Work out the finished part from the listing and answer in its coordinate system (mm). Round coordinates to 2 decimals unless told otherwise and drop trailing zeros. Order: outer loops, then holes, each group sorted by start corner. A loop starts at its lowest first (then second) coordinate and runs counter-clockwise, first axis right, second up. Notation, with made-up numbers: (68, 59.5) - (78, 59.5) arc R22 cw to (78, 84.5) - close; hole circle Ø5 at (29, -26). An arc over 180 degrees is marked (long way). One line per question, with ' | ' between items. Start each with the question number.
from build123d import *

# Parameters (mm, degrees)
SKETCH1_R                = 26.125
BOSS_EXTRUDE1_DEPTH      = 1
SKETCH2_W                = 0.65
SKETCH2_H                = 3
CUT_EXTRUDE2_DEPTH       = 38.984224
CUT_EXTRUDE2_DEPTH_BACK  = 38.984224
SKETCH3_R                = 23.625
BOSS_EXTRUDE2_DEPTH      = 13
FILLET1_R                = 1
CIRPATTERN1_COUNT        = 6
FILLET1_OF_CIRPATTERN1_R = 1


with BuildPart() as part:
    # Sketch1 → Boss-Extrude1 (new body)
    with BuildSketch(Plane(origin=(0, 0, 0), x_dir=(1, 0, 0), z_dir=(0, 1, 0))):
        with Locations(Location((0, 0, 0), (0, 0, 270))):
            Circle(SKETCH1_R)
    extrude(amount=BOSS_EXTRUDE1_DEPTH)

    # Sketch2 → Revolve1 (revolve)
    with BuildSketch(Plane.XY, mode=Mode.PRIVATE) as revolve1_sk:
        with Locations((26.45, 1.5)):
            Rectangle(SKETCH2_W, SKETCH2_H)
    revolve(revolve1_sk.sketch.rotate(Axis((0, 0, 0), (0, 1, 0)), 90), axis=Axis((0, 0, 0), (0, 1, 0)))

    # Sketch3 → Cut-Extrude2 (cut, two sides: drawn at the far end of the back side and taken through both)
    with BuildSketch(Plane(origin=(0, 0, 0), x_dir=(1, 0, 0), z_dir=(0, 1, 0)).offset(-CUT_EXTRUDE2_DEPTH_BACK)):
        with Locations(Location((0, 0, 0), (0, 0, 270))):
            Circle(SKETCH3_R)
    extrude(amount=CUT_EXTRUDE2_DEPTH + CUT_EXTRUDE2_DEPTH_BACK, mode=Mode.SUBTRACT)

    # Sketch5 → Boss-Extrude2 (add)
    with BuildSketch(Plane(origin=(0, 0, 0), x_dir=(1, 0, 0), z_dir=(0, 1, 0))):
        with BuildLine():
            Line((25.948808, 6.6), (25.318865, 6.439776))
            ThreePointArc((25.318865, 6.439776), (26.125, 0), (25.318865, -6.439776))
            Line((25.318865, -6.439776), (25.948808, -6.6))
            ThreePointArc((25.948808, -6.6), (26.775, 0), (25.948808, 6.6))
        make_face()
    boss_extrude2 = extrude(amount=BOSS_EXTRUDE2_DEPTH)

    # Fillet1
    # the kernel refuses this fillet: 1 mm, written as the material it takes off along each edge
    with BuildSketch(Plane(origin=(0, 13, 0), x_dir=(0.9431839321448116, 0, -0.33227107930701955), z_dir=(-0.33227107930701955, 0, -0.9431839321448116))) as fillet1_piece_1:
        with BuildLine():
            CenterArc((27.125, 0.93675), FILLET1_R, 180, 69.512685)
            Line((26.125, 0.93675), (26.105, 0.93675))
            Line((26.105, 0.93675), (26.105, 0))
            Line((26.105, 0), (26.125, -0.02))
            ThreePointArc((26.125, -0.02), (26.45, -0.02), (26.768, -0.018735))
            Line((26.768, -0.018735), (26.775, 0))
        make_face()
    revolve(axis=Axis((0, 13, 0), (0, -1, 0)), revolution_arc=38.813358, mode=Mode.SUBTRACT)

    # CirPattern1: Boss-Extrude2 ×6 about axis
    cirpattern1_axis = Axis((0, 0, 0), (0, 1, 0))
    for i in range(1, CIRPATTERN1_COUNT):
        add(boss_extrude2.rotate(cirpattern1_axis, i * 360 / CIRPATTERN1_COUNT))

    # Fillet1 of CirPattern1
    # the kernel refuses this fillet: 1 mm, written as the material it takes off along each edge
    with BuildSketch(Plane(origin=(0, 13, 0), x_dir=(0.18383677044965302, 0, -0.9829567853322146), z_dir=(-0.9829567853322146, 0, -0.18383677044965302))) as fillet1_of_cirpattern1_piece_1:
        with BuildLine():
            CenterArc((27.125, 0.93675), FILLET1_OF_CIRPATTERN1_R, 180, 69.512685)
            Line((26.125, 0.93675), (26.105, 0.93675))
            Line((26.105, 0.93675), (26.105, 0))
            Line((26.105, 0), (26.125, -0.02))
            ThreePointArc((26.125, -0.02), (26.45, -0.02), (26.768, -0.018735))
            Line((26.768, -0.018735), (26.775, 0))
        make_face()
    revolve(axis=Axis((0, 13, 0), (0, -1, 0)), revolution_arc=38.813358, mode=Mode.SUBTRACT)
    with BuildSketch(Plane(origin=(0, 13, 0), x_dir=(-0.7593471616951585, 0, -0.6506857060251953), z_dir=(-0.6506857060251953, 0, 0.7593471616951585))) as fillet1_of_cirpattern1_piece_2:
        with BuildLine():
            CenterArc((27.125, 0.93675), FILLET1_OF_CIRPATTERN1_R, 180, 69.512685)
            Line((26.125, 0.93675), (26.105, 0.93675))
            Line((26.105, 0.93675), (26.105, 0))
            Line((26.105, 0), (26.125, -0.02))
            ThreePointArc((26.125, -0.02), (26.45, -0.02), (26.768, -0.018735))
            Line((26.768, -0.018735), (26.775, 0))
        make_face()
    revolve(axis=Axis((0, 13, 0), (0, -1, 0)), revolution_arc=38.813358, mode=Mode.SUBTRACT)
    with BuildSketch(Plane(origin=(0, 13, 0), x_dir=(-0.9431839321448114, 0, 0.3322710793070194), z_dir=(0.3322710793070194, 0, 0.9431839321448114))) as fillet1_of_cirpattern1_piece_3:
        with BuildLine():
            CenterArc((27.125, 0.93675), FILLET1_OF_CIRPATTERN1_R, 180, 69.512685)
            Line((26.125, 0.93675), (26.105, 0.93675))
            Line((26.105, 0.93675), (26.105, 0))
            Line((26.105, 0), (26.125, -0.02))
            ThreePointArc((26.125, -0.02), (26.45, -0.02), (26.768, -0.018735))
            Line((26.768, -0.018735), (26.775, 0))
        make_face()
    revolve(axis=Axis((0, 13, 0), (0, -1, 0)), revolution_arc=38.813358, mode=Mode.SUBTRACT)
    with BuildSketch(Plane(origin=(0, 13, 0), x_dir=(-0.18383677044965369, 0, 0.9829567853322146), z_dir=(0.9829567853322146, 0, 0.18383677044965369))) as fillet1_of_cirpattern1_piece_4:
        with BuildLine():
            CenterArc((27.125, 0.93675), FILLET1_OF_CIRPATTERN1_R, 180, 69.512685)
            Line((26.125, 0.93675), (26.105, 0.93675))
            Line((26.105, 0.93675), (26.105, 0))
            Line((26.105, 0), (26.125, -0.02))
            ThreePointArc((26.125, -0.02), (26.45, -0.02), (26.768, -0.018735))
            Line((26.768, -0.018735), (26.775, 0))
        make_face()
    revolve(axis=Axis((0, 13, 0), (0, -1, 0)), revolution_arc=38.813358, mode=Mode.SUBTRACT)
    with BuildSketch(Plane(origin=(0, 13, 0), x_dir=(0.7593471616951586, 0, 0.6506857060251952), z_dir=(0.6506857060251952, 0, -0.7593471616951586))) as fillet1_of_cirpattern1_piece_5:
        with BuildLine():
            CenterArc((27.125, 0.93675), FILLET1_OF_CIRPATTERN1_R, 180, 69.512685)
            Line((26.125, 0.93675), (26.105, 0.93675))
            Line((26.105, 0.93675), (26.105, 0))
            Line((26.105, 0), (26.125, -0.02))
            ThreePointArc((26.125, -0.02), (26.45, -0.02), (26.768, -0.018735))
            Line((26.768, -0.018735), (26.775, 0))
        make_face()
    revolve(axis=Axis((0, 13, 0), (0, -1, 0)), revolution_arc=38.813358, mode=Mode.SUBTRACT)


solid = part.part
1) Section B-B on y = 5.5 is taken. Give the vertices of the cut face in (x, z) (3 decimals), and give its area (3 significant figures).
2) Section A-A on x = 0 is taken. Give the vertices of the cut face in (y, z) (3 decimals), and give its area (3 significant figures).
3) Flat-ended cylindrical pins translate along their axes: pin 1 (6 mm diameter, centred on x = 21, z = 10.5, fed in from +Y); pin 2 (6 mm diameter, centred on x = -11.5, z = 20, fed in from +Y); pin 3 (4 mm diameter, centred on x = -1.5, y = 1.5, fed in from +Z) (3 decimals). Find the tip coordinate at first contact, or state that the pin passes through.
4) Straight lines are drawn through the part: line 1 (X direction, y = 0.5, z = 0) (3 decimals); line 2 (X direction, y = 10.5, z = 0) (3 decimals); line 3 (Y direction, x = -18, z = -15.5). For each, find the intervals that lie inside material, in ascending order.
5) Section C-C on z = 0 is taken. Give the vertices of the cut face in (x, y) (3 decimals), and give its area (3 significant figures).
6) Determine the mould class of faces 1 (the cylindrical face through (-23.063, 0.493, -5.121)), 2 (the flat face through (-21, 0, 12)), 3 (the flat face through (-23.1, 1, -5.9)) for opening direction X: released by +X, released by -X, zero draft, split by the parting line, or undercut.
Recorded:
1) outline: (-25.949, -6.6) - (-25.319, -6.44) arc R26.125 cw to (-25.319, 6.44) - (-25.949, 6.6) arc R26.775 ccw to start; (-18.69, -19.172) arc R26.775 ccw to (-7.259, -25.772) - (-7.082, -25.147) arc R26.125 cw to (-18.236, -18.707) - close; (-18.69, 19.172) - (-18.236, 18.707) arc R26.125 cw to (-7.082, 25.147) - (-7.259, 25.772) arc R26.775 ccw to start; (7.082, -25.147) - (7.259, -25.772) arc R26.775 ccw to (18.69, -19.172) - (18.236, -18.707) arc R26.125 cw to start; (7.082, 25.147) arc R26.125 cw to (18.236, 18.707) - (18.69, 19.172) arc R26.775 ccw to (7.259, 25.772) - close; (25.319, -6.44) - (25.949, -6.6) arc R26.775 ccw to (25.949, 6.6) - (25.319, 6.44) arc R26.125 cw to start | area: 51.4 mm²
2) outline: (0, -26.775) - (3, -26.775) - (3, -26.125) - (1, -26.125) - (1, -23.625) - (0, -23.625) - close; (0, 23.625) - (1, 23.625) - (1, 26.125) - (3, 26.125) - (3, 26.775) - (0, 26.775) - close | area: 8.90 mm²
3) pin 1: stops at y = 3 | pin 2: stops at y = 1 | pin 3: stops at z = 26.775
4) line 1: x = -26.775 to -23.625, 23.625 to 26.775 | line 2: x = -26.775 to -26.125, 26.125 to 26.775 | line 3: y = 0 to 1
5) outline: (-26.775, 0) - (-23.625, 0) - (-23.625, 1) - (-26.125, 1) - (-26.125, 12.063) arc R1 ccw to (-26.775, 13) - close; (23.625, 0) - (26.775, 0) - (26.775, 13) arc R1 ccw to (26.125, 12.063) - (26.125, 1) - (23.625, 1) - close | area: 21.6 mm²
6) face 1: undercut | face 2: zero draft | face 3: undercut
